Check sheet for the modelled part. Datum: model origin and axes. Units: mm. A direction names the side the tool comes from. Round coordinates to 2 decimals unless told otherwise and drop trailing zeros. Write each loop counter-clockwise with the first axis right and the second up, starting at its lowest first coordinate (ties: lowest second). Pieces come first, ordered by that corner, then holes. Notation, with made-up numbers: M 55.25,-23 L 109.25,-23 A21 cw 109.25,-19 Z; hole C 2.5,85 d8. An arc over 180 degrees is marked long. Answer in a Markdown table with one row per item.
```python
from build123d import *

# Parameters (mm, degrees)
SKETCH_1_R                         = 5
SM_BASE_FLANGE_2_DEPTH             = 8
SM_EDGE_FLANGE_10_STRIP_W          = 33.4732
SM_EDGE_FLANGE_10_STRIP_H          = 8
SM_EDGE_FLANGE_10_STRIP_CUT_DEPTH  = 80
SM_EDGE_FLANGE_10_RELIEF_W         = 37.4732
SM_EDGE_FLANGE_10_RELIEF_H         = 4
SM_EDGE_FLANGE_10_RELIEF_CUT_DEPTH = 8
SM_EDGE_FLANGE_10_DEPTH            = 80
SM_EDGE_FLANGE_12_STRIP_W          = 33.4732
SM_EDGE_FLANGE_12_STRIP_H          = 8
SM_EDGE_FLANGE_12_STRIP_CUT_DEPTH  = 80
SM_EDGE_FLANGE_12_RELIEF_W         = 37.4732
SM_EDGE_FLANGE_12_RELIEF_H         = 4
SM_EDGE_FLANGE_12_RELIEF_CUT_DEPTH = 8
SM_EDGE_FLANGE_12_DEPTH            = 80


# Sheet-metal steps are written as plain solids
with BuildPart() as part:
    # 草图1 → 基体-法兰2 (new body)
    with BuildSketch(Plane.XY):
        with BuildLine():
            Line((0, 0), (80, 0))
            Line((80, 0), (80, 100))
            Line((80, 100), (58.758007847, 174.223096705))
            ThreePointArc((58.758007847, 174.223096705), (39.983985428, 180.823607775), (21.209963009, 174.223096705))
            Line((21.209963009, 174.223096705), (0, 100))
            Line((0, 100), (0, 0))
        make_face()
        with Locations((39.983985428, 150.823607775)):
            Circle(SKETCH_1_R, mode=Mode.SUBTRACT)
        with Locations((39.983985428, 130.823607775)):
            Circle(SKETCH_1_R, mode=Mode.SUBTRACT)
        with Locations((39.983985428, 110.823607775)):
            Circle(SKETCH_1_R, mode=Mode.SUBTRACT)
    extrude(amount=-SM_BASE_FLANGE_2_DEPTH)

    # 边线-法兰10 strip (across the edge) → 边线-法兰10 strip cut (cut)
    with BuildSketch(Plane(origin=(80, 80, -8), x_dir=(-1, 0, 0), z_dir=(0, -1, 0))):
        with Locations((-8, -4)):
            Rectangle(SM_EDGE_FLANGE_10_STRIP_W, SM_EDGE_FLANGE_10_STRIP_H)
    extrude(amount=SM_EDGE_FLANGE_10_STRIP_CUT_DEPTH, mode=Mode.SUBTRACT)

    # 边线-法兰10 relief (on the sheet) → 边线-法兰10 relief cut (cut)
    with BuildSketch(Plane(origin=(71.2634, 80, -8), x_dir=(-1, 0, 0), z_dir=(0, 0, -1))):
        with Locations((-14.7366, 2)):
            Rectangle(SM_EDGE_FLANGE_10_RELIEF_W, SM_EDGE_FLANGE_10_RELIEF_H)
    extrude(amount=-SM_EDGE_FLANGE_10_RELIEF_CUT_DEPTH, mode=Mode.SUBTRACT)

    # 边线-法兰10 section (across the edge) → 边线-法兰10 (add)
    with BuildSketch(Plane(origin=(80, 80, -8), x_dir=(-1, 0, 0), z_dir=(0, -1, 0))):
        with BuildLine():
            Line((0, 0.7366), (0, 72))
            Line((0, 72), (8, 72))
            Line((8, 72), (8, 0.7366))
            ThreePointArc((8, 0.7366), (8.215745145, 0.215745145), (8.7366, 0))
            Line((8.7366, 0), (8.7366, -8))
            ThreePointArc((8.7366, -8), (2.558890895, -5.441109105), (0, 0.7366))
        make_face()
    extrude(amount=SM_EDGE_FLANGE_10_DEPTH)

    # 边线-法兰12 strip (across the edge) → 边线-法兰12 strip cut (cut)
    with BuildSketch(Plane(origin=(0, 0, -8), x_dir=(1, 0, 0), z_dir=(0, 1, 0))):
        with Locations((-8, -4)):
            Rectangle(SM_EDGE_FLANGE_12_STRIP_W, SM_EDGE_FLANGE_12_STRIP_H)
    extrude(amount=SM_EDGE_FLANGE_12_STRIP_CUT_DEPTH, mode=Mode.SUBTRACT)

    # 边线-法兰12 relief (on the sheet) → 边线-法兰12 relief cut (cut)
    with BuildSketch(Plane(origin=(8.7366, 0, -8), x_dir=(1, 0, 0), z_dir=(0, 0, -1))):
        with Locations((-14.7366, -82)):
            Rectangle(SM_EDGE_FLANGE_12_RELIEF_W, SM_EDGE_FLANGE_12_RELIEF_H)
    extrude(amount=-SM_EDGE_FLANGE_12_RELIEF_CUT_DEPTH, mode=Mode.SUBTRACT)

    # 边线-法兰12 section (across the edge) → 边线-法兰12 (add)
    with BuildSketch(Plane(origin=(0, 0, -8), x_dir=(1, 0, 0), z_dir=(0, 1, 0))):
        with BuildLine():
            Line((0, 0.7366), (0, 72))
            Line((0, 72), (8, 72))
            Line((8, 72), (8, 0.7366))
            ThreePointArc((8, 0.7366), (8.215745145, 0.215745145), (8.7366, 0))
            Line((8.7366, 0), (8.7366, -8))
            ThreePointArc((8.7366, -8), (2.558890895, -5.441109105), (0, 0.7366))
        make_face()
    extrude(amount=SM_EDGE_FLANGE_12_DEPTH)


solid = part.part
```
1. Access from +Z, -Z, +X, -X, +Y, -Y to the whole of each face (thin tool, end or side, straight path). Record for faces 1 (the face through (2.63, 39.44, -2.49)), 2 (the face through (5, 80, -41)), 3 (the face through (77.37, 40.56, -2.49)), 4 (the face through (67.263, 82, -4)).
Found:
| item | result |
|---|---|
| face 1 | +Z, -X, -Y |
| face 2 | +Z, -Z, -X |
| face 3 | +Z, +X, -Y |
| face 4 | +Z, -Z, +X |
2. Section check D-D, the plane x = 50. Record the cut outline in (y, z).
Found:
| item | result |
|---|---|
| outline | M 0,-8 L 179.1,-8 L 179.1,0 L 0,0 Z |
3. Draft check along Y on faces 5 (the face through (72, 41, -45)), 6 (the face through (6, 84, -4)), 7 (the face through (40.268, 180.822, -3.944)), 8 (the face through (40.2, 0, -7.6)). Enter one of: +Y half, -Y half, draft (parallel to the pull), parting line (faces both ways), or undercut.
Found:
| item | result |
|---|---|
| face 5 | draft |
| face 6 | undercut |
| face 7 | +Y half |
| face 8 | -Y half |
4. Scan lines: L1, parallel to X at y = 26, z = -65.5; L2, parallel to Z at x = 21.5, y = 85.5; L3, parallel to Y at x = 73, z = -65.5. Record each from-to range of solid material in increasing order.
Found:
| item | result |
|---|---|
| L1 | x = 0 to 8, 72 to 80 |
| L2 | z = -8 to 0 |
| L3 | y = 0 to 80 |
5. Section check B-B, the plane y = 27. Record the cut outline in (x, z).
Found:
| item | result |
|---|---|
| outline | M 0,-80 L 8,-80 L 8,-8.74 A0.74 cw 8.74,-8 L 71.26,-8 A0.74 cw 72,-8.74 L 72,-80 L 80,-80 L 80,-8.74 A8.74 ccw 71.26,0 L 8.74,0 A8.74 ccw 0,-8.74 Z |
6. Section check C-C, the plane z = -5. Record the cut outline in (x, y), and give its area (3 significant figures).
Found:
| item | result |
|---|---|
| outline | M 0,84 L 12.74,84 L 12.74,80 L 0.84,80 L 0.84,0 L 79.16,0 L 79.16,80 L 67.26,80 L 67.26,84 L 80,84 L 80,100 L 58.76,174.22 A30 ccw 21.21,174.22 L 0,100 Z; hole C 39.98,110.82 d10; hole C 39.98,130.82 d10; hole C 39.98,150.82 d10 |
| area | 12,100 mm2 |
7. Go/stop test with flat-tipped pins: pin 1 (1.5 mm diameter, centred on x = 49, y = 144, fed in from -Z); pin 2 (4 mm diameter, centred on x = 71.5, z = -34.5, fed in from +Y). Record where each tip stops, or that it passes through.
Found:
| item | result |
|---|---|
| pin 1 | stops at z = -8 |
| pin 2 | stops at y = 80 |
8. Section check A-A, the plane z = -63. Record the cut outline in (x, y), and give its area (3 significant figures).
Found:
| item | result |
|---|---|
| outline | M 0,0 L 8,0 L 8,80 L 0,80 Z; M 72,0 L 80,0 L 80,80 L 72,80 Z |
| area | 1,280 mm2 |
